Verification items for this drawing (mm, ordinates from the low corner). A direction names the side the tool comes from. Round coordinates to 2 decimals unless told otherwise and drop trailing zeros. Write each loop counter-clockwise with the first axis right and the second up, starting at its lowest first coordinate (ties: lowest second). Pieces come first, ordered by that corner, then holes. Notation, with made-up numbers: M 59,25 L 114,25 A20 ccw 114,45 Z; hole C 59.25,84 d11. An arc over 180 degrees is marked long. One line per question, with ' | ' between items. Start each with the question number.
Q1. Gauge pin test, flat ends, axial feed: pin 1 (4.5 mm diameter, centred on x = 12.5, z = 6, fed in from +Y); pin 2 (4.5 mm diameter, centred on x = 2, z = 6.5, fed in from -Y); pin 3 (2.5 mm diameter, centred on x = 10.5, y = 3.5, fed in from +Z). Record the tip position at first contact, or that the pin passes through.
Q2. Cross-section at B-B (y = 2.5). Record the boundary of the cut face in (x, z).
Q3. Thickness scan on line 1 along X through (y, z) = (1.25, 7); line 2 along Y through (x, z) = (8, 1.2); line 3 along Z through (x, y) = (7.25, 4.1). Record the ranges inside material, lowest first. Write a range as from..to.
Q4. Cross-section at D-D (x = 9.5). Record the boundary of the cut face in (y, z).
Q5. Release check for a two-part mould opening along Y. For the marked faces 4, 5 and 6 record: released by +Y, released by -Y, zero draft, split by the parting line, or undercut.
Q6. Cross-section at A-A (z = 7). Record the boundary of the cut face in (x, y).
Q7. Cross-section at C-C (x = 13.5). Record the boundary of the cut face in (y, z), then the cut area to 3 significant figures.
Q8. Tool access check on the marked faces 1, 2 and 3. Record the directions out of +Z, -Z, +X, -X, +Y, -Y that give a thin tool (end or side, any length) a straight path to the whole face; none if there is none.
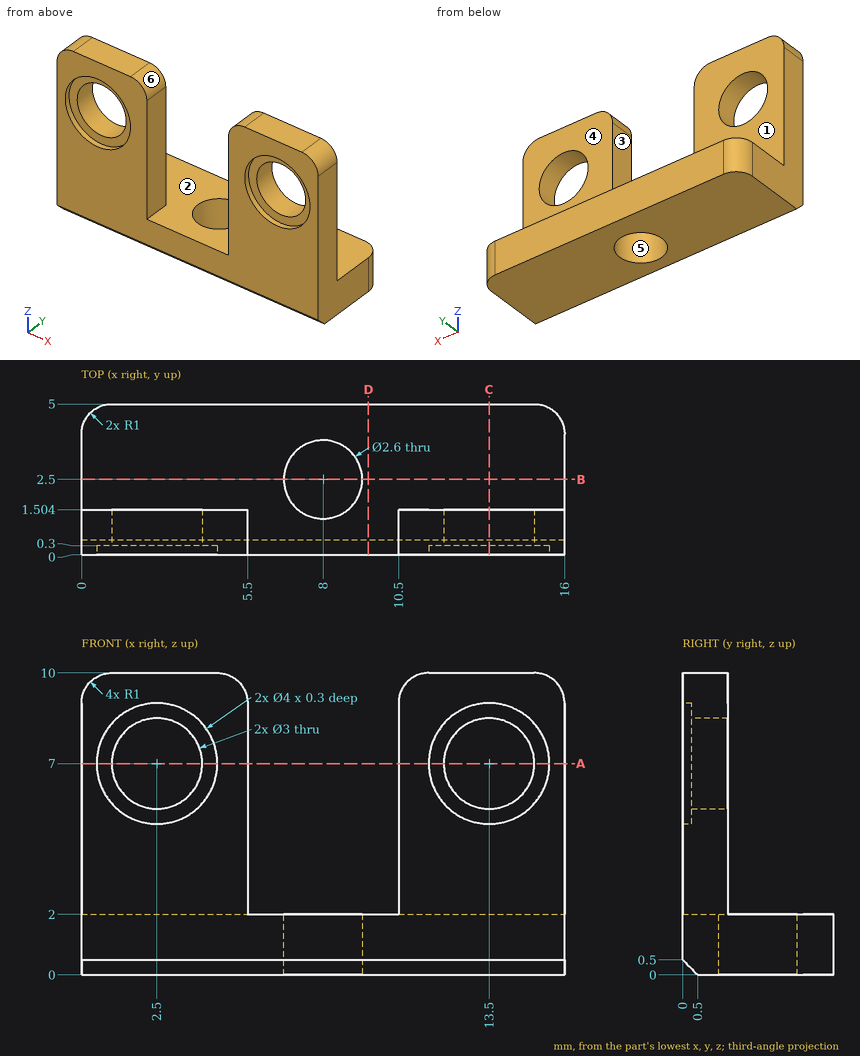
Determined:
1) pin 1: stops at y = 1.5 | pin 2: stops at y = 0 | pin 3: stops at z = 2
2) outline: M 0,0 L 6.7,0 L 6.7,2 L 0,2 Z; M 9.3,0 L 16,0 L 16,2 L 9.3,2 Z
3) line 1: x = 0..1, 4..5.5, 10.5..12, 15..16 | line 2: y = 0..1.2, 3.8..5 | line 3: z = 0..2
4) outline: M 0,0.5 L 0.5,0 L 5,0 L 5,2 L 0,2 Z
5) face 4: released by +Y | face 5: undercut | face 6: zero draft
6) outline: M 0,0 L 0.5,0 L 0.5,0.3 L 1,0.3 L 1,1.5 L 0,1.5 Z; M 4,0.3 L 4.5,0.3 L 4.5,0 L 5.5,0 L 5.5,1.5 L 4,1.5 Z; M 10.5,0 L 11.5,0 L 11.5,0.3 L 12,0.3 L 12,1.5 L 10.5,1.5 Z; M 15,0.3 L 15.5,0.3 L 15.5,0 L 16,0 L 16,1.5 L 15,1.5 Z
7) outline: M 0,0.5 L 0.5,0 L 5,0 L 5,2 L 1.5,2 L 1.5,5.5 L 0.3,5.5 L 0.3,5 L 0,5 Z; M 0,9 L 0.3,9 L 0.3,8.5 L 1.5,8.5 L 1.5,10 L 0,10 Z | area: 17.1 mm²
8) face 1: +Z, +X, -X, +Y | face 2: +Z, +Y | face 3: +Z, +Y, -Y
